Work out the finished part from the listing and answer in its coordinate system (mm). A direction names the side the tool comes from. Coordinates: 2 decimals unless noted, no trailing zeros. Order: outer loops, then holes, each group sorted by start corner. A loop starts at its lowest first (then second) coordinate and runs counter-clockwise, first axis right, second up. Notation, with made-up numbers: M 21.5,79.5 L 72.5,79.5 A24 cw 72.5,95.5 Z; hole C 30.25,-32 d5. An arc over 180 degrees is marked long. Answer in a Markdown table with one row per item. Add a question column.
Item 1: The part is cut by section A-A (x = 0). Write down the section's boundary in (y, z).
Item 2: Consider line 1 (X direction, y = -8.5, z = 16); line 2 (Y direction, x = 4, z = 9.25); line 3 (Y direction, x = 6.75, z = 10.75). Determine where each line is inside the solid, lowest interval first. Write a range as from..to.
Item 3: Flat-ended cylindrical pins translate along their axes: pin 1 Ø1 at (x, z) = (-3.5, 10) entering from +Y; pin 2 Ø5.5 at (x, y) = (0.5, 8) entering from -Z. Find the tip coordinate at first contact, or state that the pin passes through.
Item 4: The part is cut by section D-D (y = -10). Write down the section's boundary in (x, z).
Item 5: Which of the six approach directions +Z, -Z, +X, -X, +Y, -Y give full straight-line access (tool end or side, diameter ignored) to faces 1 (the face through (-8.715, -3.301, 11.577)), 2 (the face through (-2.285, -6.301, 13.098)), 3 (the face through (0, -11, 6)), 4 (the face through (0, -3, 11))?
Item 6: The mould has two halves that part along Y. Classify faces 5 (the face through (0, 11, 18)), 6 (the face through (-4, -6, 13)), 7 (the face through (0, -20, 13)), 8 (the face through (-8.715, 27.699, 18.521)): released by +Y, released by -Y, zero draft, split by the parting line, or undercut.
Item 7: The part is cut by section C-C (z = 9.25). Write down the section's boundary in (x, y).
Item 8: The part is cut by section B-B (y = 15.5). Write down the section's boundary in (x, z).
from build123d import *

# Parameters (mm, degrees)
BOX026_W          = 4
BOX026_H          = 11
BOX026_DEPTH      = 16
BOX027_W          = 4
BOX027_H          = 11
BOX027_DEPTH      = 16
FILLET004_R       = 1
BOX024_W          = 18
BOX024_H          = 17
BOX024_DEPTH      = 14
FILLET005_R       = 1
CYLINDER032_R     = 1.5
CYLINDER032_DEPTH = 10
CYLINDER033_R     = 1.5
CYLINDER033_DEPTH = 10
BOX025_W          = 3
BOX025_H          = 10
BOX025_DEPTH      = 5
BOX023_W          = 18
BOX023_H          = 32
BOX023_DEPTH      = 3
FILLET006_R       = 1


with BuildPart() as cube026:
    # Box026 → Box026 (new body)
    with BuildSketch(Plane(origin=(-6, -17, 6), x_dir=(1, 0, 0), z_dir=(0, 0, 1))):
        with Locations((2, 5.5)):
            Rectangle(BOX026_W, BOX026_H)
    extrude(amount=BOX026_DEPTH)


with BuildPart() as fillet004:
    # Box027 → Box027 (new body)
    with BuildSketch(Plane(origin=(2, -17, 6), x_dir=(1, 0, 0), z_dir=(0, 0, 1))):
        with Locations((2, 5.5)):
            Rectangle(BOX027_W, BOX027_H)
    extrude(amount=BOX027_DEPTH)

    # Fusion001001001011002004002008: union Cube026
    add(cube026.part)

    # Fillet004
    fillet004_edges = [fillet004.edges().sort_by_distance(p)[0] for p in [
        (2, -17, 14),
        (2, -6, 14),
        (6, -17, 14),
        (6, -6, 14),
        (-6, -17, 14),
        (-6, -6, 14),
        (-2, -17, 14),
        (-2, -6, 14),
    ]]
    fillet(fillet004_edges, radius=FILLET004_R)


with BuildPart() as cut002008023012009006003002006_body:
    # Box024 → Box024 (new body)
    with BuildSketch(Plane(origin=(-9, -20, 6), x_dir=(1, 0, 0), z_dir=(0, 0, 1))):
        with Locations((9, 8.5)):
            Rectangle(BOX024_W, BOX024_H)
    extrude(amount=BOX024_DEPTH)

    # Fillet005
    fillet005_edges = [cut002008023012009006003002006_body.edges().sort_by_distance(p)[0] for p in [
        (-9, -20, 13),
        (-9, -3, 13),
        (9, -20, 13),
        (9, -3, 13),
    ]]
    fillet(fillet005_edges, radius=FILLET005_R)

    # Cut002008023012009006003002006002006002004004005004: cut Fillet004
    add(fillet004.part, mode=Mode.SUBTRACT)


with BuildPart() as cylinder032:
    # Cylinder032 → Cylinder032 (new body)
    with BuildSketch(Plane(origin=(0, 12.5, 12.5), x_dir=(1, 0, 0), z_dir=(0, 0, 1))):
        Circle(CYLINDER032_R)
    extrude(amount=CYLINDER032_DEPTH)


with BuildPart() as cylinder033:
    # Cylinder033 → Cylinder033 (new body)
    with BuildSketch(Plane(origin=(0, 22.5, 12.5), x_dir=(1, 0, 0), z_dir=(0, 0, 1))):
        Circle(CYLINDER033_R)
    extrude(amount=CYLINDER033_DEPTH)


with BuildPart() as fusion001001001011002004002005:
    # Box025 → Box025 (new body)
    with BuildSketch(Plane(origin=(-1.5, 12.5, 17), x_dir=(1, 0, 0), z_dir=(0, 0, 1))):
        with Locations((1.5, 5)):
            Rectangle(BOX025_W, BOX025_H)
    extrude(amount=BOX025_DEPTH)

    # Fusion001001001011002004002005: union Cylinder032, Cylinder033
    add(cylinder032.part)
    add(cylinder033.part)


with BuildPart() as fusion001001001011002004002009:
    # Box023 → Box023 (new body)
    with BuildSketch(Plane(origin=(-9, -4, 17), x_dir=(1, 0, 0), z_dir=(0, 0, 1))):
        with Locations((9, 16)):
            Rectangle(BOX023_W, BOX023_H)
    extrude(amount=BOX023_DEPTH)

    # Cut002008023012009006003002006002006002004004005005: cut Fusion001001001011002004002005
    add(fusion001001001011002004002005.part, mode=Mode.SUBTRACT)

    # Fillet006
    fillet006_edges = [fusion001001001011002004002009.edges().sort_by_distance(p)[0] for p in [
        (-9, 28, 18.5),
        (9, 28, 18.5),
    ]]
    fillet(fillet006_edges, radius=FILLET006_R)

    # Fusion001001001011002004002009: union Cut002008023012009006003002006 body
    add(cut002008023012009006003002006_body.part)


solid = fusion001001001011002004002009.part
Reply:
| question | item | result |
|---|---|---|
| 1 | outline | M -20,6 L -3,6 L -3,17 L 11,17 L 11,20 L -20,20 Z; M 24,17 L 28,17 L 28,20 L 24,20 Z |
| 2 | line 1 | x = -9..-6, -2..2, 6..9 |
| 2 | line 2 | y = -20..-17, -6..-3 |
| 2 | line 3 | y = -20..-3 |
| 3 | pin 1 | stops at y = -3 |
| 3 | pin 2 | stops at z = 17 |
| 4 | outline | M -9,6 L -6,6 L -6,20 L -9,20 Z; M -2,6 L 2,6 L 2,20 L -2,20 Z; M 6,6 L 9,6 L 9,20 L 6,20 Z |
| 5 | face 1 | -Z, -X, +Y |
| 5 | face 2 | +Z, -Z |
| 5 | face 3 | -Z, +X, -X, +Y, -Y |
| 5 | face 4 | -Z, +X, -X, +Y |
| 6 | face 5 | undercut |
| 6 | face 6 | undercut |
| 6 | face 7 | released by -Y |
| 6 | face 8 | released by +Y |
| 7 | outline | M -9,-19 A1 ccw -8,-20 L 8,-20 A1 ccw 9,-19 L 9,-4 A1 ccw 8,-3 L -8,-3 A1 ccw -9,-4 Z; hole M -6,-16 A1 ccw -5,-17 L -3,-17 A1 ccw -2,-16 L -2,-7 A1 ccw -3,-6 L -5,-6 A1 ccw -6,-7 Z; hole M 2,-16 A1 ccw 3,-17 L 5,-17 A1 ccw 6,-16 L 6,-7 A1 ccw 5,-6 L 3,-6 A1 ccw 2,-7 Z |
| 8 | outline | M -9,17 L -1.5,17 L -1.5,20 L -9,20 Z; M 1.5,17 L 9,17 L 9,20 L 1.5,20 Z |
